Verification items for this drawing (mm, ordinates from the low corner). Coordinates: 2 decimals unless noted, no trailing zeros. Order: outer loops, then holes, each group sorted by start corner. A loop starts at its lowest first (then second) coordinate and runs counter-clockwise, first axis right, second up. Notation, with made-up numbers: (67, -10.5) - (94, -10.5) arc R12 ccw to (94, -5.5) - close; hole circle Ø2 at (4.5, 51). An arc over 180 degrees is marked (long way). Use CSV: the item, a comma, the result in double quotes. Start each with the question number.
1) Thickness scan on probe 1 along Y at (x, z) = (350, 13.5); probe 2 along X at (y, z) = (241, 32.5). Record the ranges inside material, lowest first. Write a range as [from, to].
2) Sectioned sample at B-B, the plane y = 241. Record the cut outline in (x, z), and give its area (3 significant figures).
3) Sectioned sample at A-A, the plane x = 350. Record the cut outline in (y, z).
4) Depth check by flat-ended pin: P1, Ø10, axis at x = 112, z = 7.5, coming from the -Y side. Enter the tip coordinate at first touch or a pass-through.
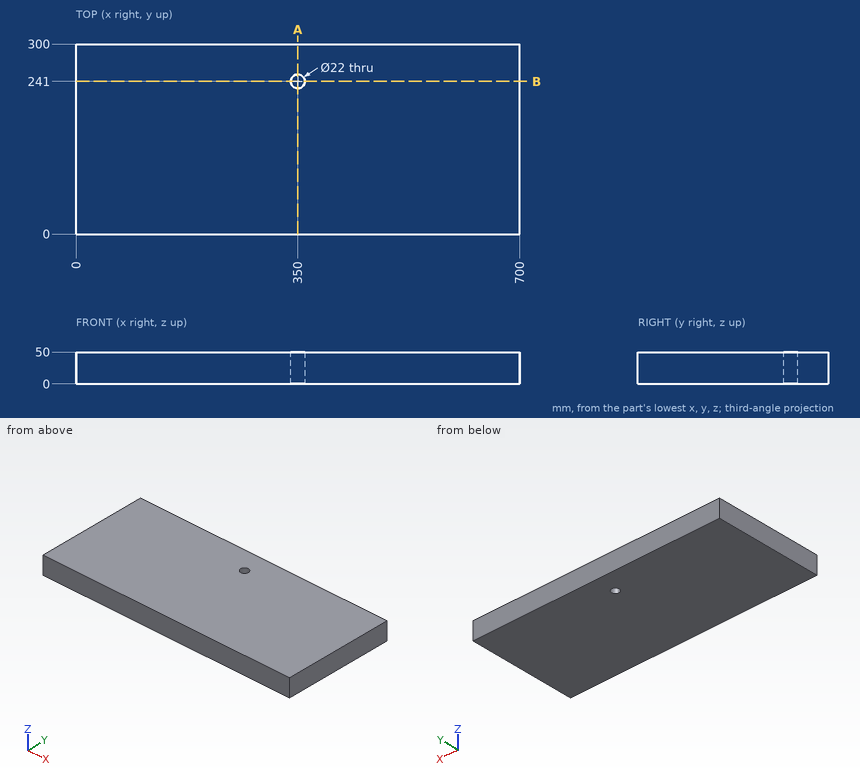
Evaluation:
1,probe 1,"[0, 230], [252, 300]"
1,probe 2,"[0, 339], [361, 700]"
2,outline,"(0, 0) - (339, 0) - (339, 50) - (0, 50) - close; (361, 0) - (700, 0) - (700, 50) - (361, 50) - close"
2,area,"33,900 mm²"
3,outline,"(0, 0) - (230, 0) - (230, 50) - (0, 50) - close; (252, 0) - (300, 0) - (300, 50) - (252, 50) - close"
4,P1,"y = 0"
